from build123d import *

# Parameters (mm, degrees)
BOSS_EXTRUDE1_DEPTH = 120
SKETCH2_R           = 2.65
CUT_EXTRUDE1_DEPTH  = 200


with BuildPart() as part:
    # Sketch1 → Boss-Extrude1 (new body)
    with BuildSketch(Plane.XY):
        Polygon((0, 0), (20, 0), (20, 45), (65, 45), (65, 0), (66, 0), (66, 46), (19, 46), (19, 1), (0, 1), align=None)
    extrude(amount=BOSS_EXTRUDE1_DEPTH)

    # Sketch2 → Cut-Extrude1 (cut)
    with BuildSketch(Plane(origin=(0, 1, 0), x_dir=(1, 0, 0), z_dir=(0, 1, 0))):
        with Locations((9.5, -30)):
            Circle(SKETCH2_R)
        with Locations((9.5, -90)):
            Circle(SKETCH2_R)
    extrude(amount=-CUT_EXTRUDE1_DEPTH, mode=Mode.SUBTRACT)


solid = part.part
Source: CAD feature listing. Evaluate the final solid. Frame: model axes, mm. A direction names the side the tool comes from. Give positions to 0.01 mm unless a question says otherwise; leave off trailing zeros. Write each loop counter-clockwise with the first axis right and the second up, starting at its lowest first coordinate (ties: lowest second). Pieces come first, ordered by that corner, then holes. Notation, with made-up numbers: (-18, 44.5) - (-8, 44.5) arc R17 cw to (-8, 59.5) - close; hole circle Ø5 at (-25.75, 18). An arc over 180 degrees is marked (long way). Write item = value, one per line. Start each with the question number.
Q1. Cut plane D-D, the plane z = 94. Return loops of the section in (x, y).
Q2. Pin query (flat end, axial travel): pin 1 Ø10 at (y, z) = (13.5, 74.5) entering from -X. Return the tip coordinate at first contact, or that it passes through.
Q3. Draft query along Z for faces 4 (the cylindrical face through (7.547, 0.507, 28.209)), 5 (the cylindrical face through (8.93, 0.51, 92.59)), 6 (the flat face through (65, 23, 59)), 7 (the flat face through (32.8, 45.3, 0)). Return one class per face: +Z half, -Z half, draft (parallel to the pull), parting line (faces both ways), or undercut.
Q4. Material intervals for probe 1 along Z at (x, y) = (9.5, 0.45); probe 2 along X at (y, z) = (0.5, 30); probe 3 along X at (y, z) = (24, 11.5), sorted ascending.
Q5. Reachability of faces 1 (the flat face through (10, 1, 59)), 2 (the flat face through (42, 45, 59)), 3 (the flat face through (43, 46, 59)) from +Z, -Z, +X, -X, +Y, -Y: full face, straight path, thin tool, end or side. Return the list, or none.
Q6. Cut plane A-A, the plane z = 30. Return loops of the section in (x, y).
Q7. Cut plane B-B, the plane y = 13. Return loops of the section in (x, z).
Q8. Cut plane C-C, the plane x = 9.5. Return loops of the section in (y, z), then the cut area to 3 significant figures.
Computed values:
q1.outline = (0, 0) - (20, 0) - (20, 45) - (65, 45) - (65, 0) - (66, 0) - (66, 46) - (19, 46) - (19, 1) - (0, 1) - close
q2.pin_1 = 19
q3.face_4 = undercut
q3.face_5 = undercut
q3.face_6 = draft
q3.face_7 = -Z half
q4.probe_1 = 0 to 27.35, 32.65 to 87.35, 92.65 to 120
q4.probe_2 = 0 to 6.85, 12.15 to 20, 65 to 66
q4.probe_3 = 19 to 20, 65 to 66
q5.face_1 = +Z, -Z, -X, +Y
q5.face_2 = +Z, -Z, -Y
q5.face_3 = +Z, -Z, +X, -X, +Y
q6.outline = (0, 0) - (6.85, 0) - (6.85, 1) - (0, 1) - close; (12.15, 0) - (20, 0) - (20, 45) - (65, 45) - (65, 0) - (66, 0) - (66, 46) - (19, 46) - (19, 1) - (12.15, 1) - close
q7.outline = (19, 0) - (20, 0) - (20, 120) - (19, 120) - close; (65, 0) - (66, 0) - (66, 120) - (65, 120) - close
q8.outline = (0, 0) - (1, 0) - (1, 27.35) - (0, 27.35) - close; (0, 32.65) - (1, 32.65) - (1, 87.35) - (0, 87.35) - close; (0, 92.65) - (1, 92.65) - (1, 120) - (0, 120) - close
q8.area = 109 mm²
